For this review, take the finished solid that the model builds, in its own axes (mm). Face numbers are marked on the shaded views. Round coordinates to 2 decimals unless told otherwise and drop trailing zeros. Loops run counter-clockwise (first coordinate to the right, second up) from the corner with the lowest first, then second, coordinate; pieces in that order, holes last.
1) Wall thickness on L1, parallel to X at y = 6.25, z = -11.25; L2, parallel to X at y = 4.5, z = -12.5; L3, parallel to Z at x = 28.5, y = 4: over which ranges is each line inside the solid? List them lowest first.
2) Insertion check: pin 1 (1.8 mm diameter, centred on x = 14.5, z = -11.95, fed in from +Y); pin 2 (3 mm diameter, centred on x = 13, z = -6, fed in from +Y); pin 3 (3 mm diameter, centred on x = 36, z = -17, fed in from +Y). Each pin has a flat end and moves straight along its axis. Give the tip position at first contact, or say it passes through.
3) Take a section at B-B (x = 40). State the section outline as (y, z) points.
4) Take a section at A-A (x = 14.5). State the section outline as (y, z) points, then the cut area to 3 significant figures.
5) Mouldability with a two-part tool opening along Z and no side actions: class the marked faces 1, 2, 3 and 4 as pulls with the +Z half, pulls with the -Z half, needs draft (parallel to the pull), parting line crosses it, or undercut.
6) Take a section at C-C (y = 3.5). State the section outline as (x, z) points.
7) Take a section at D-D (y = 5.75). State the section outline as (x, z) points.
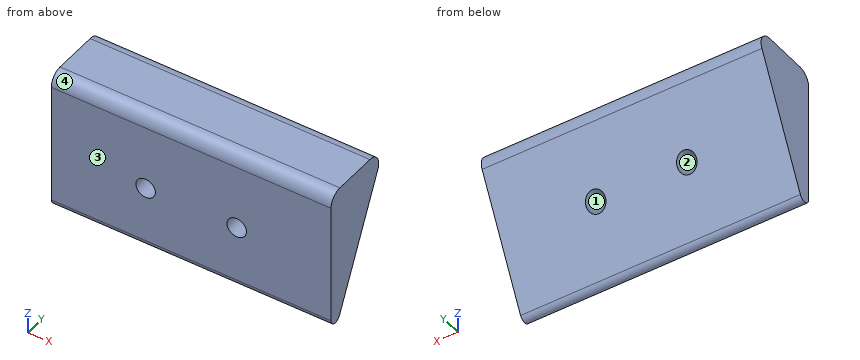
```python
from build123d import *

# Parameters (mm, degrees)
BOSS_EXTRUDE1_DEPTH = 43
SKETCH2_R           = 1.5
CUT_EXTRUDE1_DEPTH  = 50.150879706


with BuildPart() as part:
    # Sketch1 → Boss-Extrude1 (new body)
    with BuildSketch(Plane(origin=(0, 0, 0), x_dir=(0, 0, -1), z_dir=(1, 0, 0))):
        with BuildLine():
            Line((2, 0), (20.605762563, 0))
            ThreePointArc((20.605762563, 0), (21.580832575, 0.778102566), (21.03849363, 1.901523057))
            Line((21.03849363, 1.901523057), (2.865462135, 10.624578175))
            ThreePointArc((2.865462135, 10.624578175), (0.934853125, 10.514299657), (0, 8.82153206))
            Line((0, 8.82153206), (0, 2))
            ThreePointArc((0, 2), (0.585786438, 0.585786438), (2, 0))
        make_face()
    extrude(amount=BOSS_EXTRUDE1_DEPTH)

    # Sketch2 → Cut-Extrude1 (cut, through all)
    with BuildSketch(Plane(origin=(0, 10, 0), x_dir=(1, 0, 0), z_dir=(0, 1, 0))):
        with Locations(Location((14.5, 11.951977883, 0), (0, 0, 270))):
            Circle(SKETCH2_R)
        with Locations(Location((28.5, 11.951977883, 0), (0, 0, 270))):
            Circle(SKETCH2_R)
    extrude(amount=-CUT_EXTRUDE1_DEPTH, mode=Mode.SUBTRACT)


solid = part.part
```
Response:
1. L1: x = 0 to 13.17, 15.83 to 27.17, 29.83 to 43
1. L2: x = 0 to 13.1, 15.9 to 27.1, 29.9 to 43
1. L3: z = -16.67 to -13.45, -10.45 to 0
2. pin 1: passes through
2. pin 2: stops at y = 9.84
2. pin 3: stops at y = 4.56
3. outline: (0, -20.61) arc R1 ccw to (1.9, -21.04) - (10.62, -2.87) arc R2 ccw to (8.82, 0) - (2, 0) arc R2 ccw to (0, -2) - close
4. outline: (0, -20.61) arc R1 ccw to (1.9, -21.04) - (5.54, -13.45) - (0, -13.45) - close; (0, -10.45) - (6.98, -10.45) - (10.62, -2.87) arc R2 ccw to (8.82, 0) - (2, 0) arc R2 ccw to (0, -2) - close
4. area: 125 mm2
5. face 1: undercut
5. face 2: undercut
5. face 3: needs draft
5. face 4: pulls with the +Z half
6. outline: (0, -17.71) - (43, -17.71) - (43, 0) - (0, 0) - close; hole circle Ø3 at (14.5, -11.95); hole circle Ø3 at (28.5, -11.95)
7. outline: (0, -13.02) - (13.45, -13.02) arc R1.5 cw (long way) to (15.55, -13.02) - (27.45, -13.02) arc R1.5 cw (long way) to (29.55, -13.02) - (43, -13.02) - (43, 0) - (0, 0) - close
